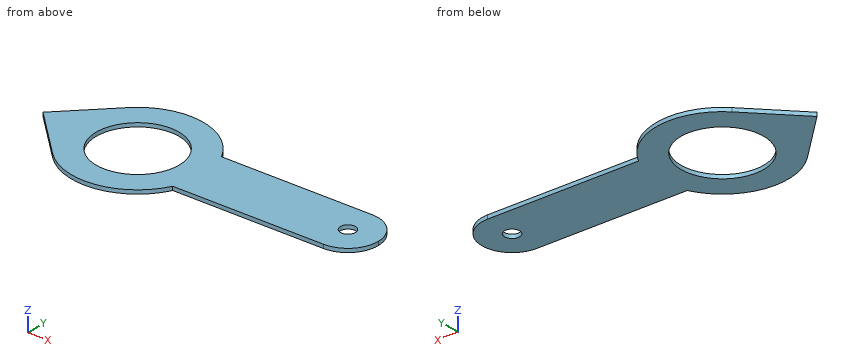
```python
from build123d import *

# Parameters (mm, degrees)
F0_R     = 11
F0_R_2   = 2
F1_DEPTH = 1


with BuildPart() as f1:
    # F0 (on Top) → F1 (new body)
    with BuildSketch(Plane.XY):
        with BuildLine():
            ThreePointArc((-37.5, 0), (-37.990786, 4.115417), (-39.435618, 8))
            ThreePointArc((-39.435618, 8), (-52.293005, 17.289366), (-67.374369, 12.374369))
            ThreePointArc((-67.374369, 12.374369), (-72.5, 0), (-67.374369, -12.374369))
            ThreePointArc((-67.374369, -12.374369), (-52.293005, -17.289366), (-39.435618, -8))
            ThreePointArc((-39.435618, -8), (-37.990786, -4.115417), (-37.5, 0))
        make_face()
        with Locations((-55, 0)):
            Circle(F0_R, mode=Mode.SUBTRACT)
        with BuildLine():
            ThreePointArc((-67.374369, -12.374369), (-72.5, 0), (-67.374369, 12.374369))
            Line((-67.374369, 12.374369), (-79.748737, 0))
            Line((-79.748737, 0), (-67.374369, -12.374369))
        make_face()
        with BuildLine():
            ThreePointArc((0, -8), (-8, 0), (0, 8))
            Line((0, 8), (-39.435618, 8))
            ThreePointArc((-39.435618, 8), (-37.990786, 4.115417), (-37.5, 0))
            ThreePointArc((-37.5, 0), (-37.990786, -4.115417), (-39.435618, -8))
            Line((-39.435618, -8), (0, -8))
        make_face()
        with BuildLine():
            ThreePointArc((0, -8), (5.656854, -5.656854), (8, 0))
            ThreePointArc((8, 0), (5.656854, 5.656854), (0, 8))
            ThreePointArc((0, 8), (-8, 0), (0, -8))
        make_face()
        Circle(F0_R_2, mode=Mode.SUBTRACT)
    extrude(amount=F1_DEPTH)


solid = f1.part
```
The model under review builds one solid part; all positions refer to its coordinate system, in mm. Round coordinates to 2 decimals unless told otherwise and drop trailing zeros. Order: outer loops, then holes, each group sorted by start corner. A loop starts at its lowest first (then second) coordinate and runs counter-clockwise, first axis right, second up.
(1) Take a section at B-B, the plane x = -55. State the section outline as (y, z) points.
Working result:
outline: (-17.5, 0) - (-11, 0) - (-11, 1) - (-17.5, 1) - close; (11, 0) - (17.5, 0) - (17.5, 1) - (11, 1) - close
(2) Wall thickness on L1, parallel to Y at x = 0, z = 0.8; L2, parallel to Y at x = -55, z = 0.45; L3, parallel to X at y = -4, z = 0.6: over which ranges is each line inside the solid? List them lowest first.
Working result:
L1: y = -8 to -2, 2 to 8
L2: y = -17.5 to -11, 11 to 17.5
L3: x = -75.75 to -65.25, -44.75 to 6.93
(3) Take a section at C-C, the plane y = 4. State the section outline as (x, z) points, plus the area to 3 significant figures.
Working result:
outline: (-75.75, 0) - (-65.25, 0) - (-65.25, 1) - (-75.75, 1) - close; (-44.75, 0) - (6.93, 0) - (6.93, 1) - (-44.75, 1) - close
area: 62.2 mm2
(4) For P1, Ø1.5, axis at x = -15.5, y = -8, coming from the -Z side, flat-tipped, find the tip position at first contact; note if it passes through.
Working result:
P1: stops at z = 0
(5) Take a section at D-D, the plane x = -8.5. State the section outline as (y, z) points, plus the area to 3 significant figures.
Working result:
outline: (-8, 0) - (8, 0) - (8, 1) - (-8, 1) - close
area: 16.0 mm2
(6) Take a section at A-A, the plane z = 0.65. State the section outline as (x, y) points, plus the area to 3 significant figures.
Working result:
outline: (-79.75, 0) - (-67.37, -12.37) arc R17.5 ccw to (-39.44, -8) - (0, -8) arc R8 ccw to (8, 0) arc R8 ccw to (0, 8) - (-39.44, 8) arc R17.5 ccw to (-67.37, 12.37) - close; hole circle Ø22 at (-55, 0); hole circle Ø4 at (0, 0)
area: 1,350 mm2
